Verification items for this drawing (mm, ordinates from the low corner). A direction names the side the tool comes from. Coordinates: 2 decimals unless noted, no trailing zeros. Loops run counter-clockwise (first coordinate to the right, second up) from the corner with the lowest first, then second, coordinate; pieces in that order, holes last. Notation, with made-up numbers: M 33.5,-18 L 56.5,-18 A12 cw 56.5,-5 Z; hole C 40.25,23.5 d9. An arc over 180 degrees is marked long. Return JSON: item names as keys, results as strings.
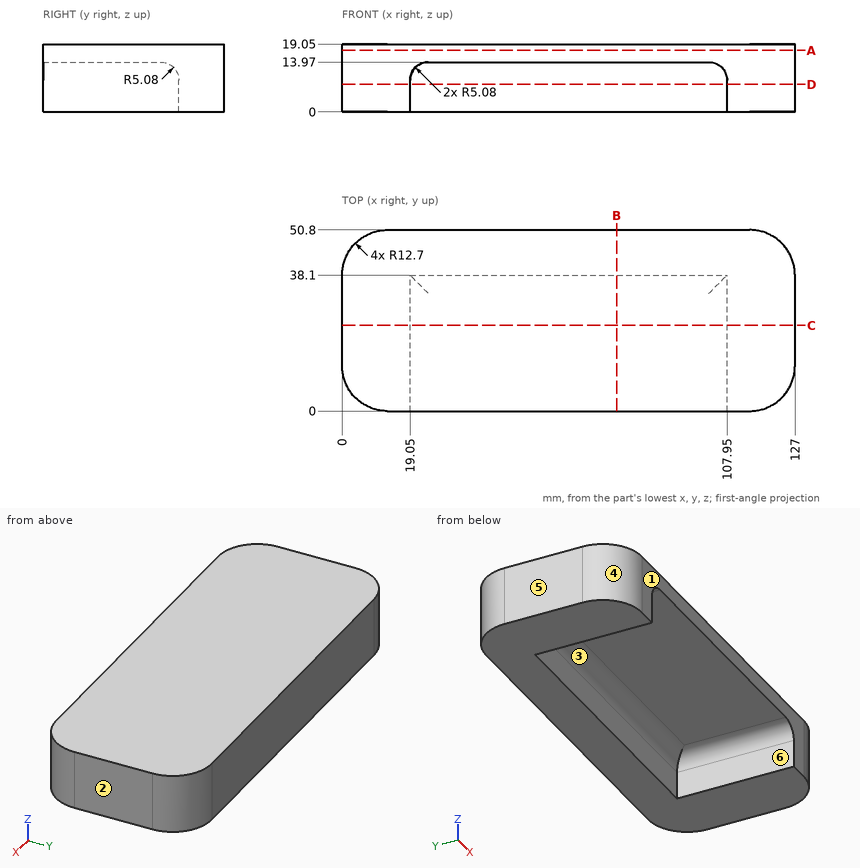
1) Section check C-C on y = 24. Record the cut outline in (x, z), then the cut area to 3 significant figures.
Answers:
{"outline": "M 0,0 L 19.05,0 L 19.05,8.89 A5.08 cw 24.13,13.97 L 102.87,13.97 A5.08 cw 107.95,8.89 L 107.95,0 L 127,0 L 127,19.05 L 0,19.05 Z", "area": "1,190 mm²"}
2) Scan lines: line 1 along X through (y, z) = (32, 1); line 2 along Z through (x, y) = (61.5, 7); line 3 along X through (y, z) = (32, 12.5). Record each from-to range of solid material in increasing order. Write a range as [from, to].
Answers:
{"line 1": "[0, 19.05], [107.95, 127]", "line 2": "[13.97, 19.05]", "line 3": "[0, 20.56], [106.44, 127]"}
3) Section check A-A on z = 17.25. Record the cut outline in (x, y).
Answers:
{"outline": "M 0,12.7 A12.7 ccw 12.7,0 L 114.3,0 A12.7 ccw 127,12.7 L 127,38.1 A12.7 ccw 114.3,50.8 L 12.7,50.8 A12.7 ccw 0,38.1 Z"}
4) Go/stop test with flat-tipped pins: pin 1 Ø3 at (x, y) = (103, 9.5) entering from -Z; pin 2 Ø6 at (y, z) = (5.5, 15) entering from -X; pin 3 Ø10 at (x, z) = (71.5, 2.5) entering from -Y. Record where each tip stops, or that it passes through.
Answers:
{"pin 1": "z = 13.7", "pin 2": "x = 0.71", "pin 3": "y = 38.1"}
5) Draft check along X on the marked faces 1, 2, 3 and 4. Enter one of: +X half, -X half, draft (parallel to the pull), parting line (faces both ways), or undercut.
Answers:
{"face 1": "draft", "face 2": "+X half", "face 3": "undercut", "face 4": "-X half"}
6) Set-up check for the marked faces 5 and 6: record each of +Z, -Z, +X, -X, +Y, -Y from which the full face is reachable in a straight line by a thin tool's end or side.
Answers:
{"face 5": "+Z, -Z, -X, +Y, -Y", "face 6": "-Z, -Y"}
7) Section check D-D on z = 7.75. Record the cut outline in (x, y), then the cut area to 3 significant figures.
Answers:
{"outline": "M 0,12.7 A12.7 ccw 12.7,0 L 19.05,0 L 19.05,38.1 L 107.95,38.1 L 107.95,0 L 114.3,0 A12.7 ccw 127,12.7 L 127,38.1 A12.7 ccw 114.3,50.8 L 12.7,50.8 A12.7 ccw 0,38.1 Z", "area": "2,930 mm²"}
8) Section check B-B on x = 77. Record the cut outline in (y, z).
Answers:
{"outline": "M 0,13.97 L 33.02,13.97 A5.08 cw 38.1,8.89 L 38.1,0 L 50.8,0 L 50.8,19.05 L 0,19.05 Z"}
